Autodesk Inventor part; units mm, degrees
ref_plane "YZ Plane" through (0, 0, 0) normal (1, 0, 0) x (0, 1, 0)
ref_plane "XZ Plane" through (0, 0, 0) normal (0, 1, 0) x (-1, 0, 0)
ref_plane "XY Plane" through (0, 0, 0) normal (0, 0, 1) x (1, 0, 0)
sketch "Sketch1" plane through (0, 0, 0) normal (1, 0, 0) x (0, 1, 0)
  line L0 (0, 0) -> (0, 11)
  line L1 (0, 11) -> (0, 11)
  line L2 (0, 11) -> (25, 1.9007)
  line L3 (25, 1.9007) -> (25, 0)
  line L4 (25, 0) -> (0, 0)
  dimension "d0" = 11
  dimension "d1" = 160
  dimension "d2" = 25
  dimension "d4" = 0
extrude "Extrusion1" add sketch "Sketch1" along normal blind 8
sketch "Sketch2" plane through (0, 0, 0) normal (0, -1, 0) x (1, 0, 0)
  circle A0 centre (4, 5) radius 4
  line L0 (0, 11) -> (0, 0)
  line L1 (8, 11) -> (8, 0)
  line L2 (0, 0) -> (8, 0)
  circle A1 centre (4, 5) radius 3.125
  circle A2 centre (4, 5) radius 1.5
  line L3 (0, 11) -> (8, 11)
  dimension "d7" = 6.25
  dimension "d8" = 3
  dimension "d21" = 6
extrude "Extrusion2" cut sketch "Sketch2" against normal through all contours A2
extrude "Extrusion3" cut sketch "Sketch2" against normal blind 4.25 contours A1
extrude "Extrusion4" add sketch "Sketch2" along normal blind 1 contours A0
sketch "Sketch3" plane through (0, 25, 1.9007) normal (0, 1, 0) x (1, 0, 0)
  circle A0 centre (4, -3.0993) radius 2.5
  circle A1 centre (4, -3.0993) radius 1.5
  point P0 (0, 1.9007)
  dimension "d15" = 5
extrude "Extrusion5" cut sketch "Sketch3" against normal blind 19.75 contours A0 | A1
sketch "Sketch5" plane through (0, 0, 11) normal (0, -1, 0) x (1, 0, 0)
  arc A0 (8, -6) -> (0, -6) centre (4, -6) ccw
  line L0 (8, 0) -> (8, -6)
  line L1 (0, 0) -> (8, 0)
  line L2 (0, 0) -> (0, -6)
  point P0 (0, -11)
extrude "Extrusion7" add sketch "Sketch5" along normal up to surface (1 mm away)
fillet "Fillet2" radius 5 1 edges at (4, 0, 11)
properties part number "rpi_stand"
Can you work these out from the model? Positions are in its coordinate system, mm. A direction names the side the tool comes from. Give positions to 0.01 mm unless a question says otherwise; leave off trailing zeros. Order: outer loops, then holes, each group sorted by start corner. A loop starts at its lowest first (then second) coordinate and runs counter-clockwise, first axis right, second up. Notation, with made-up numbers: (43.25, 53) - (72.25, 53) arc R20 ccw to (72.25, 57) - close; hole circle Ø5 at (-2, 64.25). An arc over 180 degrees is marked (long way). Use a Markdown table: item, result. Add a question column.
Q1. I'm going to push flat-ended pins straight in: pin 1 (1.9 mm diameter, centred on x = 5, z = 4.5, fed in from -Y); pin 2 (4 mm diameter, centred on x = 4, z = 5, fed in from +Y). Where does each tip first touch, or does it pass through?
Q2. Please list where these lines run through material, in increasing order: line 1 along Z through (x, y) = (4, 10.5); line 2 along Z through (x, y) = (4, 5.05); line 3 along X through (y, z) = (9, 4.25).
Q3. If we section it at B-B on x = 5: Write out the boundary of the cut face in (y, z).
Q4. If we section it at D-D on x = 2.25: Write out the boundary of the cut face in (y, z).
Q5. If we mould it in two halves opening along X, with no side actions, what happens to faces 1 (the flat face through (4, 13, 0)), 2 (the cylindrical face through (4.1, -0.5, 1)), 3 (the cylindrical face through (3.67, 12.43, 2.52))? For each: released by +X, released by -X, zero draft, split by the parting line, or undercut.
Q6. If we section it at C-C on y = 9.5: Write out the boundary of the cut face in (x, z), plus the area to 3 significant figures.
Q7. On a 3-axis mill with a long thin cutter (end or side, diameter ignored), from which of +Z, -Z, +X, -X, +Y, -Y can I reach the whole of each face in a straight line? I mean faces 4 (the flat face through (6, 5.25, 5)), 5 (the cylindrical face through (1.52, 1.66, 6.9)), 6 (the flat face through (3.9, 0, 0.8)). Say none if no direction works.
Answers follow:
| question | item | result |
|---|---|---|
| 1 | pin 1 | stops at y = 4.25 |
| 1 | pin 2 | stops at y = 5.25 |
| 2 | line 1 | z = 0 to 2.5 |
| 2 | line 2 | z = 0 to 3.5, 6.5 to 9.16 |
| 2 | line 3 | x = 0 to 1.62, 6.38 to 8 |
| 3 | outline | (-1, 1.13) - (0, 1.13) - (0, 0) - (25, 0) - (25, 1.9) - (22.78, 2.71) - (5.25, 2.71) - (5.25, 3.88) - (4.25, 3.88) - (4.25, 2.04) - (-1, 2.04) - close; (-1, 7.96) - (4.25, 7.96) - (4.25, 6.12) - (5.25, 6.12) - (5.25, 7.29) - (10.19, 7.29) - (0.83, 10.7) arc R5 ccw to (-0.88, 11) - (-1, 11) - close |
| 4 | outline | (-1, 1.4) - (0, 1.4) - (0, 0) - (25, 0) - (25, 1.9) - (21.39, 3.21) - (5.25, 3.21) - (5.25, 6.79) - (11.58, 6.79) - (0.83, 10.7) arc R5 ccw to (-0.88, 11) - (-1, 11) - (-1, 7.59) - (4.25, 7.59) - (4.25, 2.41) - (-1, 2.41) - close |
| 5 | face 1 | zero draft |
| 5 | face 2 | split by the parting line |
| 5 | face 3 | undercut |
| 6 | outline | (0, 0) - (8, 0) - (8, 7.54) - (0, 7.54) - close; hole circle Ø5 at (4, 5) |
| 6 | area | 40.7 mm^2 |
| 7 | face 4 | +Y |
| 7 | face 5 | -Y |
| 7 | face 6 | -Z, -Y |
